Autodesk Inventor part; units mm, degrees
ref_plane "YZ Plane" through (0, 0, 0) normal (1, 0, 0) x (0, 1, 0)
ref_plane "XZ Plane" through (0, 0, 0) normal (0, 1, 0) x (-1, 0, 0)
ref_plane "XY Plane" through (0, 0, 0) normal (0, 0, 1) x (1, 0, 0)
sketch "Sketch1" plane through (0, 0, 0) normal (0, 0, 1) x (1, 0, 0)
  line L0 (0, 0) -> (13.925, 0)
  line L1 (13.925, 0) -> (13.925, 11.5)
  line L2 (13.925, 11.5) -> (0, 11.5)
  line L3 (0, 11.5) -> (0, 0)
  line L4 (0, 0) -> (2.5, 0)
  line L5 (2.5, 0) -> (2.5, 25.4)
  line L6 (2.5, 25.4) -> (0, 25.4)
  line L7 (0, 25.4) -> (0, 0)
  line L8 (0, 0) -> (17.5, 0)
  line L9 (17.5, 0) -> (17.5, 19.05)
  line L10 (17.5, 19.05) -> (0, 19.05)
  line L11 (0, 19.05) -> (0, 0)
  line L12 (13.925, 11.5) -> (12.5, 11.5)
  line L13 (12.5, 11.5) -> (12.5, 7.5)
  line L14 (12.5, 7.5) -> (13.925, 7.5)
  line L15 (13.925, 7.5) -> (13.925, 11.5)
  point P0 (2.5, 19.05)
  point P1 (2.5, 11.5)
  point P2 (13.925, 0)
  dimension "d0" = 13.925
  dimension "d1" = 11.5
  dimension "d2" = 2.5
  dimension "d3" = 25.4
  dimension "d4" = 17.5
  dimension "d5" = 19.05
  dimension "d6" = 4
  dimension "d7" = 12.5
revolve "Revolution1" add sketch "Sketch1" angle 360 about axis through (0, 19.05, 0) along (0, -1, 0) contours L1 L2 L5 L10 L9 L8
chamfer "Chamfer1" distance 3.175 angle 45 1 edges at (-17.5, 19.05, 0)
chamfer "Chamfer2" distance 0.5 angle 45 3 edges at (-13.925, 0, 0) (-2.5, 11.5, 0) (-2.5, 19.05, 0)
properties part number "Flywheel" material "Brass, Soft Yellow"
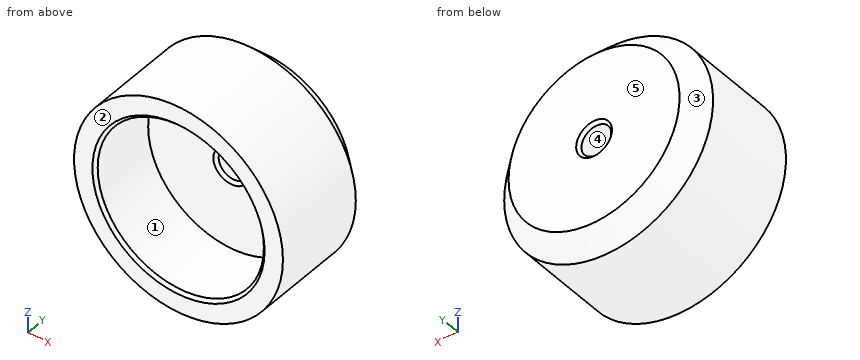
Geometry check sheet. Reference: the model listing, model coordinates, mm. Face numbers are marked on the shaded views. A direction names the side the tool comes from. Round coordinates to 2 decimals unless told otherwise and drop trailing zeros. Loops run counter-clockwise (first coordinate to the right, second up) from the corner with the lowest first, then second, coordinate; pieces in that order, holes last. Notation, with made-up numbers: (89, -20) - (110, -20) arc R26 ccw to (110, 16) - close; hole circle Ø3 at (-34, -12). An arc over 180 degrees is marked (long way). Use a Markdown table: item, result.
Q1. Material ranges on line 1 (Z direction, x = 0, y = 14.5); line 2 (Y direction, x = -9, z = -10); line 3 (Z direction, x = -4, y = 1), recorded low to high.
Solutions:
| item | result |
|---|---|
| line 1 | z = -17.5 to -2.5, 2.5 to 17.5 |
| line 2 | y = 11.5 to 19.05 |
| line 3 | z = -17.04 to -13.34, 13.34 to 17.04 |
Q2. Cross-section at C-C on y = 1. Record the cut outline in (x, z) (3 decimals), plus the area to 3 significant figures.
Solutions:
| item | result |
|---|---|
| outline | circle Ø35 at (0, 0); hole circle Ø27.85 at (0, 0) |
| area | 353 mm2 |
Q3. Cross-section at B-B on x = 0. Record the cut outline in (y, z) (3 decimals), plus the area to 3 significant figures.
Solutions:
| item | result |
|---|---|
| outline | (0, -17.5) - (15.875, -17.5) - (19.05, -14.325) - (19.05, -3) - (18.55, -2.5) - (12, -2.5) - (11.5, -3) - (11.5, -13.925) - (0.5, -13.925) - (0, -14.425) - close; (0, 14.425) - (0.5, 13.925) - (11.5, 13.925) - (11.5, 3) - (12, 2.5) - (18.55, 2.5) - (19.05, 3) - (19.05, 14.325) - (15.875, 17.5) - (0, 17.5) - close |
| area | 298 mm2 |
Q4. Draft check along Z on the marked faces 3, 4 and 5. Enter one of: released by +Z, released by -Z, zero draft, split by the parting line, or undercut.
Solutions:
| item | result |
|---|---|
| face 3 | split by the parting line |
| face 4 | undercut |
| face 5 | zero draft |
Q5. Cross-section at A-A on z = 0. Record the cut outline in (x, y) (3 decimals).
Solutions:
| item | result |
|---|---|
| outline | (-17.5, 0) - (-14.425, 0) - (-13.925, 0.5) - (-13.925, 11.5) - (-3, 11.5) - (-2.5, 12) - (-2.5, 18.55) - (-3, 19.05) - (-14.325, 19.05) - (-17.5, 15.875) - close; (2.5, 12) - (3, 11.5) - (13.925, 11.5) - (13.925, 0.5) - (14.425, 0) - (17.5, 0) - (17.5, 15.875) - (14.325, 19.05) - (3, 19.05) - (2.5, 18.55) - close |
Q6. Access from +Z, -Z, +X, -X, +Y, -Y to the whole of each face (thin tool, end or side, straight path). Record for the marked faces 1 and 2.
Solutions:
| item | result |
|---|---|
| face 1 | -Y |
| face 2 | +Z, -Z, +X, -X, -Y |
Q7. Go/stop test with flat-tipped pins: P1, Ø1.5, axis at y = 11.5, z = 6, coming from the -X side; P2, Ø4, axis at x = -8.5, y = 16, coming from the +Z side; P3, Ø5, axis at y = 2.5, z = 3.5, coming from the -X side. Record where each tip stops, or that it passes through.
Solutions:
| item | result |
|---|---|
| P1 | stops at x = -16.69 |
| P2 | stops at z = 16.25 |
| P3 | stops at x = -17.47 |
